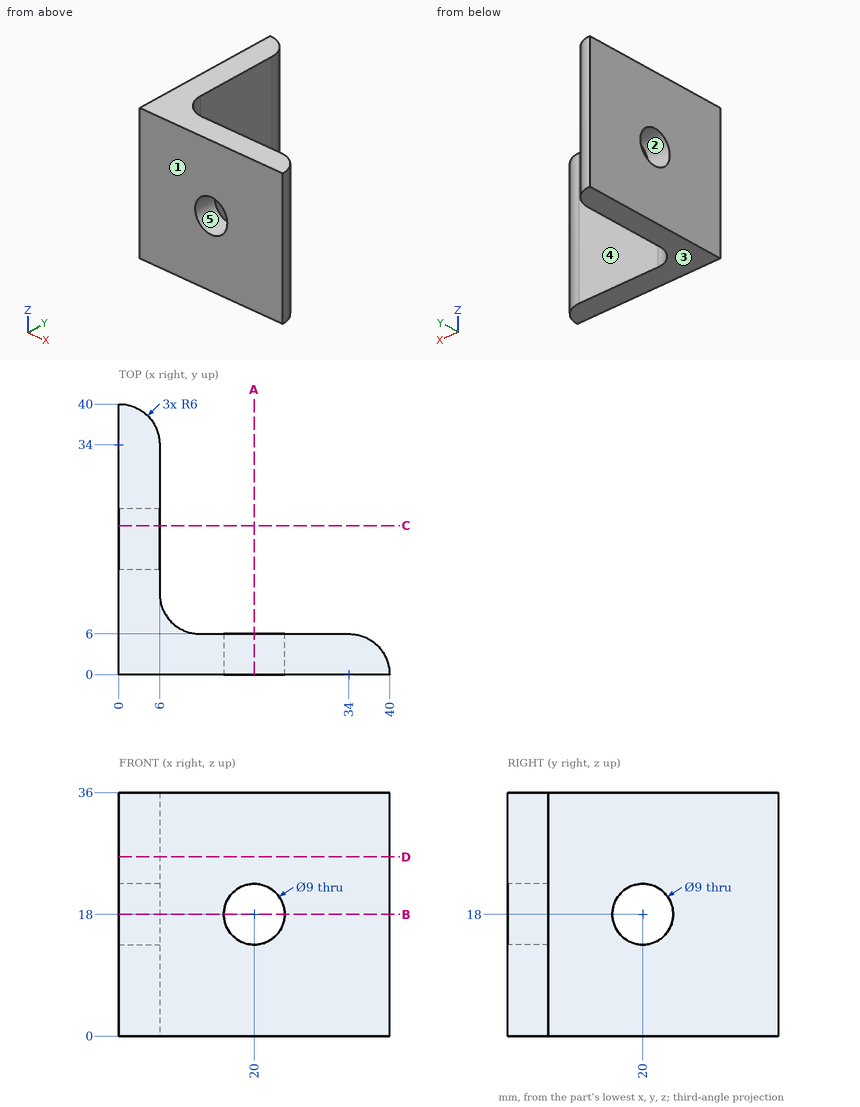
Design review of the part shown in the three views and the two pictorial views. Dimensions are in mm from the part's minimum x, y and z. A direction names the side the tool comes from. Round coordinates to 2 decimals unless told otherwise and drop trailing zeros. Order: outer loops, then holes, each group sorted by start corner. A loop starts at its lowest first (then second) coordinate and runs counter-clockwise, first axis right, second up. Notation, with made-up numbers: M -30,-4 L -7,-4 A21 ccw -7,3 Z; hole C 39,24 d9. An arc over 180 degrees is marked long. Put each result on its own line as item: value.
Q1. Insertion check: pin 1 Ø1.5 at (y, z) = (31.5, 16.5) entering from +X; pin 2 Ø4 at (x, z) = (23.5, 15.5) entering from +Y; pin 3 Ø5 at (x, y) = (12, 8) entering from +Z. Each pin has a flat end and moves straight along its axis. Give the tip position at first contact, or say it passes through.
Reported:
pin 1: x = 6
pin 2: y = 6
pin 3: z = 36
Q2. Consider section D-D (z = 26.5). State the section outline as (x, y) points, and give its area (3 significant figures).
Reported:
outline: M 0,0 L 40,0 A6 ccw 34,6 L 12,6 A6 cw 6,12 L 6,34 A6 ccw 0,40 Z
area: 436 mm²
Q3. Machinability: for the marked faces 4 and 5, which of the approach directions +Z, -Z, +X, -X, +Y, -Y give a long, thin tool a straight path to every point of the face, cutting with its end or side? Answer none if there is none.
Reported:
face 4: +Z, -Z, +X, +Y
face 5: +Y, -Y
Q4. Consider section C-C (y = 22). State the section outline as (x, z) points, and give its area (3 significant figures).
Reported:
outline: M 0,0 L 6,0 L 6,13.97 L 0,13.97 Z; M 0,22.03 L 6,22.03 L 6,36 L 0,36 Z
area: 168 mm²
Q5. Consider section B-B (z = 18). State the section outline as (x, y) points, and give its area (3 significant figures).
Reported:
outline: M 0,0 L 15.5,0 L 15.5,6 L 12,6 A6 cw 6,12 L 6,15.5 L 0,15.5 Z; M 0,24.5 L 6,24.5 L 6,34 A6 ccw 0,40 Z; M 24.5,0 L 40,0 A6 ccw 34,6 L 24.5,6 Z
area: 328 mm²
Q6. Consider section A-A (x = 20). State the section outline as (y, z) points, and give its area (3 significant figures).
Reported:
outline: M 0,0 L 6,0 L 6,13.5 L 0,13.5 Z; M 0,22.5 L 6,22.5 L 6,36 L 0,36 Z
area: 162 mm²
Q7. To check wall thickness, follow line 1 (Z direction, x = 20, y = 3.5); line 2 (X direction, y = 15.5, z = 10.5). State the ranges of each line that lie inside material, in increasing order.
Reported:
line 1: 0 to 13.5, 22.5 to 36
line 2: 0 to 6
Q8. Draft analysis for pull direction Y (two halves, no side actions). For the marked faces 1, 2 and 3, state which applies: released by +Y, released by -Y, zero draft, split by the parting line, or undercut.
Reported:
face 1: released by -Y
face 2: undercut
face 3: zero draft
